Check sheet for the modelled part. Datum: model origin and axes. Units: mm. A direction names the side the tool comes from. Round coordinates to 2 decimals unless told otherwise and drop trailing zeros. Write each loop counter-clockwise with the first axis right and the second up, starting at its lowest first coordinate (ties: lowest second). Pieces come first, ordered by that corner, then holes. Notation, with made-up numbers: M 59,-9.5 L 79,-9.5 A18 ccw 79,8.5 Z; hole C 3.25,58 d6. An arc over 180 degrees is marked long. One line per item, written item: value.
Autodesk Fusion 360 part; units mm, degrees
sketch "Sketch2" plane through (0, 0, 0) normal (0, 0, 1) x (-1, 0, 0)
  line L0 (-34, 24) -> (-34, -24)
  line L1 (-34, -24) -> (34, -24)
  line L2 (34, -24) -> (34, 24)
  line L3 (34, 24) -> (-34, 24)
  line L4 (34.1, 24.1) -> (-34.1, 24.1)
  line L5 (-34.1, 24.1) -> (-34.1, -24.1)
  line L6 (-34.1, -24.1) -> (34.1, -24.1)
  line L7 (34.1, -24.1) -> (34.1, 24.1)
  line L8 (34.1, 24.1) -> (-34.1, -24.1) construction
  line L9 (-34.1, 24.1) -> (34.1, -24.1) construction
  dimension "d5" = 68.2
  dimension "d6" = 48.2
extrude "Extrude2" add sketch "Sketch2" along normal blind 5 contours L0 L1 L2 L3 | L4 L5 L6 L7
shell "Shell1" thickness 4 removed faces 2 at (11.3667, 8.0333, 0) at (11.3667, 8.0333, 5)
sketch "pillar sketch" plane through (0, 0, 5) normal (0, 0, 1) x (-1, 0, 0)
  line L0 (30.1, -20.1) -> (-30.1, -20.1)
  line L1 (-30.1, -20.1) -> (-30.1, 20.1)
  line L2 (-30.1, 20.1) -> (30.1, 20.1)
  line L3 (30.1, 20.1) -> (30.1, -20.1)
  line L4 (34.1, -24.1) -> (34.1, 24.1)
  line L5 (34.1, 24.1) -> (-34.1, 24.1)
  line L6 (-34.1, 24.1) -> (-34.1, -24.1)
  line L7 (-34.1, -24.1) -> (34.1, -24.1)
  circle A0 centre (0, 19.9) radius 2.1
  circle A1 centre (29.9, 10) radius 2.1
  circle A2 centre (-29.9, 10) radius 2.1
  circle A3 centre (20, -19.9) radius 2.1
  circle A4 centre (-20, -19.9) radius 2.1
  dimension "d11" = 4.2
  dimension "d15" = 4.2
  dimension "d18" = 4.2
  dimension "d23" = 0.2
  dimension "d24" = 0.2
  dimension "d25" = 0.2
  dimension "d27" = 4.2
  dimension "d28" = 0.2
  dimension "d29" = 10.1
  dimension "d30" = 10.1
  dimension "d31" = 10.1
  dimension "d32" = 4.2
  dimension "d33" = 0.2
  dimension "d34" = 10.1
extrude "Extrude3" add sketch "pillar sketch" against normal blind 5 contours L0 A3 | L3 A1 | L0 A4 | L2 A0 | L1 A2 picked at (20.5146, -19.3943) picked at (30.7031, 10.2036) picked at (-19.3838, -19.1714) picked at (0.1862, 20.8048) picked at (-29.3932, 10.2832)
sketch "hollow sketch A" plane through (0, 0, 5) normal (0, 0, 1) x (-1, 0, 0)
  line L0 (30.1, -20.1) -> (22.0905, -20.1)
  arc A0 (22.0905, -20.1) -> (17.9095, -20.1) centre (20, -19.9) ccw
  line L1 (17.9095, -20.1) -> (-17.9095, -20.1)
  arc A1 (-17.9095, -20.1) -> (-22.0905, -20.1) centre (-20, -19.9) ccw
  line L2 (-22.0905, -20.1) -> (-30.1, -20.1)
  line L3 (-30.1, -20.1) -> (-30.1, 7.9095)
  arc A2 (-30.1, 7.9095) -> (-30.1, 12.0905) centre (-29.9, 10) ccw
  line L4 (-30.1, 12.0905) -> (-30.1, 20.1)
  line L5 (-30.1, 20.1) -> (-2.0905, 20.1)
  arc A3 (-2.0905, 20.1) -> (2.0905, 20.1) centre (0, 19.9) ccw
  line L6 (2.0905, 20.1) -> (30.1, 20.1)
  line L7 (30.1, 20.1) -> (30.1, 12.0905)
  arc A4 (30.1, 12.0905) -> (30.1, 7.9095) centre (29.9, 10) ccw
  line L8 (30.1, 7.9095) -> (30.1, -20.1)
  line L9 (34.1, -24.1) -> (34.1, 24.1)
  line L10 (34.1, 24.1) -> (-34.1, 24.1)
  line L11 (-34.1, 24.1) -> (-34.1, -24.1)
  line L12 (-34.1, -24.1) -> (34.1, -24.1)
  circle A5 centre (20, 20.3) radius 2.1
  circle A6 centre (30.3, -10) radius 2.1
  circle A7 centre (-30.3, -10) radius 2.1
  circle A8 centre (0, -20.3) radius 2.1
  circle A9 centre (-20, 20.3) radius 2.1
  dimension "d37" = 4.2
  dimension "d38" = 4.2
  dimension "d39" = 4.2
  dimension "d40" = 4.2
  dimension "d41" = 4.2
  dimension "d42" = 0.2
  dimension "d44" = 0.2
  dimension "d45" = 10.1
  dimension "d46" = 10.1
  dimension "d47" = 10.1
  dimension "d49" = 10.1
  dimension "d51" = 0.2
extrude "Extrude4" add sketch "hollow sketch A" against normal blind 3 from surface at -2 contours L8 A6 | L1 A8 | L6 A5 | L3 A7 | L5 A9 picked at (30.8398, -9.8081) picked at (-0.308, -21.7247) picked at (20.5114, 18.7272) picked at (-28.7439, -10.2036) picked at (-20.6202, 19.3298)
extrude "Extrude5" cut sketch "hollow sketch A" against normal blind 2 contours L8 A6 | L1 A8 | L1 A8 | L6 A5 | L6 A5 | L3 A7 | L3 A7 | L5 A9 | L5 A9 picked at (30.8398, -9.8081)
equation "d5 = 68 mm + space_error * 2"
equation "d6 = 48 mm + space_error * 2"
equation "error_hollow = 0.2 mm"
equation "d11 = diam_pillar"
equation "diam_hollow = 4.2 mm"
equation "error_pillar = 0.2 mm"
equation "diam_pillar = 4.2 mm"
equation "d15 = diam_pillar"
equation "d18 = diam_pillar"
equation "d23 = error_pillar"
equation "d24 = error_pillar"
equation "d25 = error_pillar"
equation "d27 = diam_pillar"
equation "d28 = error_pillar"
equation "d29 = 10 mm + space_error"
equation "d30 = 10 mm + space_error"
equation "d31 = 10 mm + space_error"
equation "d32 = diam_pillar"
equation "d33 = error_pillar"
equation "d34 = 10 mm + space_error"
equation "d37 = diam_hollow"
equation "d38 = diam_hollow"
equation "d39 = diam_hollow"
equation "d40 = diam_hollow"
equation "d41 = diam_hollow"
equation "d42 = error_hollow"
equation "d44 = error_hollow"
equation "d45 = 10 mm + space_error"
equation "d46 = 10 mm + space_error"
equation "d47 = 10 mm + space_error"
equation "space_error = 0.1 mm"
equation "d49 = 10 mm + space_error"
equation "d51 = error_hollow"
Q1. Sectioned sample at A-A on y = 6.5. Enter the section's corners in (x, z).
Completed:
outline: M -34.1,0 L -30.1,0 L -30.1,5 L -34.1,5 Z; M 30.1,0 L 34.1,0 L 34.1,5 L 30.1,5 Z
Q2. Sectioned sample at C-C on z = 1.5. Enter the section's corners in (x, y).
Completed:
outline: M -34.1,-24.1 L 34.1,-24.1 L 34.1,24.1 L -34.1,24.1 Z; hole M -30.1,-20.1 L -22.09,-20.1 A2.1 cw -17.91,-20.1 L 17.91,-20.1 A2.1 cw 22.09,-20.1 L 30.1,-20.1 L 30.1,-12.09 A2.1 cw long 30.1,-7.91 L 30.1,7.91 A2.1 cw 30.1,12.09 L 30.1,20.1 L 22.09,20.1 A2.1 cw long 17.91,20.1 L -17.91,20.1 A2.1 cw long -22.09,20.1 L -30.1,20.1 Z
Q3. Draft check along X on faces 4 (the cylindrical face through (28.2, 10, 1.5)), 5 (the flat face through (34.1, 0, 2)), 6 (the flat face through (0, -24.1, 2)). Enter one of: pulls with the +X half, pulls with the -X half, needs draft (parallel to the pull), parting line crosses it, or undercut.
Completed:
face 4: undercut
face 5: pulls with the +X half
face 6: needs draft
Q4. Scan lines: line 1 (X direction, y = -20.3, z = 3.65); line 2 (Y direction, x = -2, z = 1.5); line 3 (X direction, y = 20, z = 3.75). Record each from-to range of solid material in increasing order. Write a range as [from, to].
Completed:
line 1: [-34.1, -22.1], [-17.9, 17.9], [22.1, 34.1]
line 2: [-24.1, -20.1], [20.1, 24.1]
line 3: [-34.1, -30.1], [-22.1, -17.9], [17.9, 22.1], [30.1, 34.1]
Q5. Depth check by flat-ended pin: P1, Ø3.5, axis at x = -30.3, y = 10, coming from the +Z side; P2, Ø1.8, axis at x = -31.5, y = 10.5, coming from the +Z side. Enter the tip coordinate at first touch or a pass-through.
Completed:
P1: z = 3
P2: z = 5
Q6. Access from +Z, -Z, +X, -X, +Y, -Y to the whole of each face (thin tool, end or side, straight path). Record for faces 1 (the flat face through (0, -22, 0)), 2 (the flat face through (0, 21, 3)), 3 (the flat face through (-30.1, 0, 2)).
Completed:
face 1: -Z, +X, -X, +Y, -Y
face 2: +Z
face 3: +Z, -Z
Q7. Sectioned sample at B-B on x = -24.5. Enter the section's corners in (y, z).
Completed:
outline: M -24.1,0 L -20.1,0 L -20.1,5 L -24.1,5 Z; M 20.1,0 L 24.1,0 L 24.1,5 L 20.1,5 Z
